from build123d import *

# Parameters (mm, degrees)
F0_W     = 5
F0_H     = 28
F1_DEPTH = 14
F3_DEPTH = 18
F4_R     = 2.5
F5_DEPTH = 5
F6_R     = 2


# Not quite as in the source:
# - a feature names something its author has since deleted; it is built from what else it names


with BuildPart() as f1:
    # F0 (on Front) → F1 (new body, symmetric)
    with BuildSketch(Plane.XZ):
        Polygon((3.75, 8.5), (-6.25, 8.5), (-6.25, 6.5), (-1.25, 6.5), (3.75, 6.5), align=None)
        with Locations((1.25, -7.5)):
            Rectangle(F0_W, F0_H)
    extrude(amount=F1_DEPTH, both=True)

    # F2 (on face) → F3 (join)
    with BuildSketch(Plane.XY.offset(8.5)):
        with BuildLine():
            Line((-1.9743843018, 14.4904378137), (-3.7243843018, 14.4904378137))
            Line((-3.7243843018, 14.4904378137), (-0.1705003797, 10.7404378137))
            Line((-0.1705003797, 10.7404378137), (-4.1205003797, 6.5904378137))
            Line((-4.1205003797, 6.5904378137), (-0.1705003797, 2.8404378137))
            Line((-0.1705003797, 2.8404378137), (-4.1205003797, -1.3095621863))
            Line((-4.1205003797, -1.3095621863), (-0.1705003797, -5.0595621863))
            Line((-0.1705003797, -5.0595621863), (-4.1205003797, -9.2095621863))
            Line((-4.1205003797, -9.2095621863), (0.4322179562, -13.2100868422))
            ThreePointArc((0.4322179562, -13.2100868422), (0.838165637, -12.8418212057), (1.1682262547, -12.4042448269))
            Line((1.1682262547, -12.4042448269), (-2.3705003797, -9.2095621863))
            Line((-2.3705003797, -9.2095621863), (1.5794996203, -5.0595621863))
            Line((1.5794996203, -5.0595621863), (-2.3705003797, -1.3095621863))
            Line((-2.3705003797, -1.3095621863), (1.5794996203, 2.8404378137))
            Line((1.5794996203, 2.8404378137), (-2.3705003797, 6.5904378137))
            Line((-2.3705003797, 6.5904378137), (1.5794996203, 10.7404378137))
            Line((1.5794996203, 10.7404378137), (-1.9743843018, 14.4904378137))
        make_face()
    extrude(amount=F3_DEPTH)

    # F4 (on face) → F5 (cut, symmetric)
    with BuildSketch(Plane(origin=(-1.25, 0, 0), x_dir=(0, -1, 0), z_dir=(-1, 0, 0))):
        with Locations((8.4821127024, -15.6142489255)):
            Circle(F4_R)
    extrude(amount=F5_DEPTH, both=True, mode=Mode.SUBTRACT)

    # F6
    f6_edges = [f1.edges().sort_by_distance(p)[0] for p in [
        (3.75, -5.982113, -15.614249),
        (-1.25, -5.982113, -15.614249),
    ]]
    fillet(f6_edges, radius=F6_R)


solid = f1.part
Here's how the part is built. I have some questions about the finished solid (model axes, mm). A direction names the side the tool comes from. Round coordinates to 2 decimals unless told otherwise and drop trailing zeros. Order: outer loops, then holes, each group sorted by start corner. A loop starts at its lowest first (then second) coordinate and runs counter-clockwise, first axis right, second up. Notation, with made-up numbers: M 27.5,-9.75 L 46.5,-9.75 A21 cw 46.5,21.25 Z; hole C -14.75,77.5 d6. An arc over 180 degrees is marked long. Return JSON: item names as keys, results as strings. Group by question number.
1. On a 3-axis mill with a long thin cutter (end or side, diameter ignored), from which of +Z, -Z, +X, -X, +Y, -Y can I reach the whole of each face in a straight line? I mean faces 4 (the face through (-2.12, 8.69, 17.37)), 5 (the face through (-4, 0, 6.5)), 6 (the face through (1.24, -9.83, -13.51)), 7 (the face through (0, 0, 8.5)), 8 (the face through (-0.37, 4.69, 17.37)). Say none if no direction works.
2. I'm going to push flat-ended pins straight in: pin 1 Ø14 at (y, z) = (6.5, -3.5) entering from -X; pin 2 Ø3 at (x, z) = (0.5, -6) entering from +Y; pin 3 Ø1 at (x, y) = (-2, 2) entering from +Z; pin 4 Ø4 at (y, z) = (-8.48, -15.61) entering from +X. Where does each tip first touch, or does it pass through?
3. If we section it at C-C on z = -1.5: List the corners of the cut face in (x, y) for me.
4. If we section it at A-A on z = 12: List the corners of the cut face in (x, y) for me.
5. Please list where these lines run through material, in increasing order: probe 1 along Y at (x, z) = (-3.5, 24.5); probe 2 along X at (y, z) = (-5.5, -19); probe 3 along Z at (x, y) = (3, 10.5).
6. If we mould it in two halves opening along Y, with no side actions, what happens to faces 1 (the face through (-1.88, -11.18, 17.37)), 2 (the face through (-0.42, -7.16, 17.37)), 3 (the face through (-1.25, 0, -8))? For each: pulls with the +Y half, pulls with the -Y half, needs draft (parallel to the pull), parting line crosses it, or undercut.
7. If we section it at B-B on y = 2: List the corners of the cut face in (x, z) for me, then the cut area to 4 significant figures.
8. If we section it at D-D on z = 7: List the corners of the cut face in (x, y) for me.
Reply:
{
 "1": {"face 4": "+Z, -X", "face 5": "-Z, -X, +Y, -Y", "face 6": "+X, -X", "face 7": "+Z", "face 8": "+Z, +X"},
 "2": {"pin 1": "x = -1.25", "pin 2": "y = 14", "pin 3": "z = 8.5", "pin 4": "through"},
 "3": {"outline": "M -1.25,-14 L 3.75,-14 L 3.75,14 L -1.25,14 Z"},
 "4": {"outline": "M -4.12,-9.21 L 0.43,-13.21 A2.92 ccw 1.17,-12.4 L -2.37,-9.21 L 1.58,-5.06 L -2.37,-1.31 L 1.58,2.84 L -2.37,6.59 L 1.58,10.74 L -1.97,14.49 L -3.72,14.49 L -0.17,10.74 L -4.12,6.59 L -0.17,2.84 L -4.12,-1.31 L -0.17,-5.06 Z"},
 "5": {"probe 1": "-9.75 to -8.56, -1.9 to -0.66, 6 to 7.24, 14.25 to 14.49", "probe 2": "-1.25 to 3.75", "probe 3": "-21.5 to 8.5"},
 "6": {"face 1": "pulls with the -Y half", "face 2": "undercut", "face 3": "needs draft"},
 "7": {"outline": "M -6.25,6.5 L -1.25,6.5 L -1.25,-21.5 L 3.75,-21.5 L 3.75,8.5 L 0.78,8.5 L 0.78,26.5 L -0.97,26.5 L -0.97,8.5 L -6.25,8.5 Z", "area": "191.5 mm^2"},
 "8": {"outline": "M -6.25,-14 L 3.75,-14 L 3.75,14 L -6.25,14 Z"}
}
